Autodesk Inventor part; units mm, degrees
ref_plane "YZ Plane" through (0, 0, 0) normal (1, 0, 0) x (0, 1, 0)
ref_plane "XZ Plane" through (0, 0, 0) normal (0, 1, 0) x (-1, 0, 0)
ref_plane "XY Plane" through (0, 0, 0) normal (0, 0, 1) x (1, 0, 0)
sketch "Sketch1" plane through (0, 0, 0) normal (0, 1, 0) x (-1, 0, 0)
  circle A0 centre (0, 0) radius 32.5
  line L0 (0, 32.5) -> (0, 102.5)
  line L1 (0, 102.5) -> (0, 169.7)
  circle A1 centre (0, 136.1) radius 33.6
  circle A2 centre (0, 136.1) radius 42.65
  line L2 (42.65, 136.1) -> (40.15, 136.1)
  line L3 (40.15, 136.1) -> (62.55, 136.1)
  circle A3 centre (62.55, 136.1) radius 22.4
  line L4 (62.55, 136.1) -> (62.55, 134.2)
  line L5 (62.55, 136.1) -> (62.55, 138)
  circle A4 centre (62.55, 136.1) radius 2.8
  line L6 (62.55, 138) -> (64.6067, 138)
  line L7 (62.55, 138) -> (60.4933, 138)
  line L8 (62.55, 134.2) -> (60.4933, 134.2)
  line L9 (62.55, 134.2) -> (64.6067, 134.2)
  circle A5 centre (62.55, 136.1) radius 4.7
  line L10 (0, -32.5) -> (0, -37.5)
  circle A6 centre (0, 0) radius 37.5
  line L11 (0, 32.5) -> (5, 32.5)
  line L12 (5, 32.5) -> (5, 93.7441)
  line L13 (0, 32.5) -> (-5, 32.5)
  line L14 (-5, 32.5) -> (-5, 93.7441)
  line L15 (0, 0) -> (29.257, 0) construction
  line L16 (0, 0) -> (37.5, 0) construction
  line L17 (0, 0) -> (32.476, 18.75)
  line L18 (0, 0) -> (37.5, 0) construction
  line L19 (0, 0) -> (-32.476, 18.75)
  line L20 (0, 0) -> (37.5, 0) construction
  line L21 (0, 169.7) -> (0, 174.7)
  circle A7 centre (0, 136.1) radius 38.6
  line L22 (67.25, 136.1) -> (69.25, 136.1)
  line L23 (62.55, 140.8) -> (62.55, 142.8)
  line L24 (62.55, 131.4) -> (62.55, 129.4)
  line L25 (5, 93.7441) -> (5, 102.8741)
  line L26 (-5, 93.7441) -> (-5, 102.8741)
  line L27 (62.55, 129.4) -> (32.9252, 129.4)
  line L28 (62.55, 142.8) -> (32.9252, 142.8)
  line L29 (62.55, 142.8) -> (69.25, 142.8)
  line L30 (69.25, 142.8) -> (69.25, 136.1)
  line L31 (69.25, 129.4) -> (69.25, 136.1)
  line L32 (69.25, 129.4) -> (62.55, 129.4)
  line L33 (0, 136.1) -> (-18.0247, 97.446)
  line L34 (0, 136.1) -> (42.65, 136.1) construction
  line L35 (0, 136.1) -> (-18.0247, 174.754)
  line L36 (0, 136.1) -> (42.65, 136.1) construction
  point P0 (37.3613, 126.4)
  point P1 (41.8047, 144.5494)
  point P2 (41.8047, 127.6506)
  point P3 (42.1205, 129.4)
  point P4 (42.1205, 142.8)
  point P5 (5, 97.8252)
  point P6 (38.0141, 129.4)
  point P7 (41.1755, 129.4)
  point P8 (41.1755, 142.8)
  point P9 (38.0141, 142.8)
  point P10 (-5, 97.8252)
  point P11 (-16.3131, 171.0835)
  point P12 (-14.2, 166.5519)
  point P13 (-14.2, 105.6481)
  point P14 (-16.3131, 101.1165)
  dimension "d0" = 65
  dimension "d1" = 70
  dimension "d2" = 67.2
  dimension "d3" = 85.3
  dimension "d4" = 2.5
  dimension "d6" = 22.4
  dimension "d7" = 1.9
  dimension "d8" = 1.9
  dimension "d9" = 5.6
  dimension "d10" = 9.4
  dimension "d11" = 5
  dimension "d12" = 5
  dimension "d13" = 5
  dimension "d16" = 30
  dimension "d17" = 150
  dimension "d18" = 5
  dimension "d19" = 2
  dimension "d20" = 2
  dimension "d21" = 2
  dimension "d28" = 115
  dimension "d29" = 115
extrude "Extrusion1" add sketch "Sketch1" along normal blind 6 contours A7 L26 A1 L0 | L0 A1 L25 A7 | A7 L33 A1 L26 | L25 A1 L27 A7 | L27 A3 L2 A2 | A2 L3 A5 L24 L27 | L27 A7 L28 A3 | L27 A1 L28 A7 | A7 L21 A1 L35 | L2 A3 L28 A2 | A2 L28 L23 A5 L3 | L24 A5 L22 L31 L32 | L21 A7 L28 A1 | A5 | L29 L30 L22 A5 L23
chamfer "Chamfer1" distance 2 angle 45 1 edges at (-59.75, 0, 136.1)
fillet "Fillet1" radius 2 4 edges at (-69.25, 3, 129.4) (-69.25, 3, 142.8) (16.3131, 3, 101.1165) (16.3131, 3, 171.0835)
properties part number "door mount backplate"
Check sheet for the modelled part. Datum: model origin and axes. Units: mm. A direction names the side the tool comes from. Round coordinates to 2 decimals unless told otherwise and drop trailing zeros. Order: outer loops, then holes, each group sorted by start corner. A loop starts at its lowest first (then second) coordinate and runs counter-clockwise, first axis right, second up.
Q1. Cross-section at D-D, the plane x = 0. Enter the section's corners in (y, z), plus the area to 3 significant figures.
Filled sheet:
outline: (0, 97.5) - (6, 97.5) - (6, 102.5) - (0, 102.5) - close; (0, 169.7) - (6, 169.7) - (6, 174.7) - (0, 174.7) - close
area: 60.0 mm2
Q2. Cross-section at C-C, the plane x = -62.55. Enter the section's corners in (y, z).
Filled sheet:
outline: (0, 129.4) - (6, 129.4) - (6, 133.3) - (2, 133.3) - (0, 131.3) - close; (0, 140.9) - (2, 138.9) - (6, 138.9) - (6, 142.8) - (0, 142.8) - close
Q3. Cross-section at A-A, the plane y = 1.1. Enter the section's corners in (x, z), plus the area to 3 significant figures.
Filled sheet:
outline: (-69.25, 131.4) arc R2 ccw to (-67.25, 129.4) - (-38.01, 129.4) arc R38.6 ccw to (14.38, 100.28) arc R2 ccw to (15.44, 102.98) - (14.2, 105.65) arc R33.6 cw (long way) to (14.2, 166.55) - (15.44, 169.22) arc R2 ccw to (14.38, 171.92) arc R38.6 ccw to (-38.01, 142.8) - (-67.25, 142.8) arc R2 ccw to (-69.25, 140.8) - close; hole circle Ø7.4 at (-62.55, 136.1)
area: 1,090 mm2
Q4. Set-up check for faces 1 (the face through (14.814, 2.958, 104.332)), 2 (the face through (-33.587, 2.958, 137.044)), 3 (the face through (-53, 3, 129.4)): record each of +Z, -Z, +X, -X, +Y, -Y from which the full face is reachable in a straight line by a thin tool's end or side.
Filled sheet:
face 1: +X, +Y, -Y
face 2: +Y, -Y
face 3: -Z, -X, +Y, -Y
Q5. Cross-section at B-B, the plane z = 136.1. Enter the section's corners in (x, y), plus the area to 3 significant figures.
Filled sheet:
outline: (-69.25, 0) - (-67.35, 0) - (-65.35, 2) - (-65.35, 6) - (-69.25, 6) - close; (-59.75, 2) - (-57.75, 0) - (-33.6, 0) - (-33.6, 6) - (-59.75, 6) - close
area: 176 mm2
Q6. Scan lines: L1, parallel to X at y = 2.45, z = 136.1; L2, parallel to Z at x = 0, y = 4.15; L3, parallel to Z at x = -62.55, y = 3.45. Record each from-to range of solid material in increasing order.
Filled sheet:
L1: x = -69.25 to -65.35, -59.75 to -33.6
L2: z = 97.5 to 102.5, 169.7 to 174.7
L3: z = 129.4 to 133.3, 138.9 to 142.8
Q7. Draft check along Z on faces 4 (the face through (-62.185, 3.972, 133.324)), 5 (the face through (-53, 3, 142.8)), 6 (the face through (-64.123, 1.875, 133.634)), 7 (the face through (-69.25, 3, 136)). Enter one of: pulls with the +Z half, pulls with the -Z half, needs draft (parallel to the pull), parting line crosses it, or undercut.
Filled sheet:
face 4: undercut
face 5: pulls with the +Z half
face 6: undercut
face 7: needs draft
Q8. Depth check by flat-ended pin: P1, Ø5, axis at x = -62.55, z = 136.1, coming from the -Y side; P2, Ø3, axis at x = -18.5, y = 3, coming from the +Z side; P3, Ø3, axis at x = -59, y = 2, coming from the +Z side; P4, Ø3, axis at x = -37, y = 1.5, coming from the +Z side. Enter the tip coordinate at first touch or a pass-through.
Filled sheet:
P1: passes through
P2: stops at z = 170.75
P3: stops at z = 142.8
P4: stops at z = 151.26
